```python
from build123d import *

# Parameters (mm, degrees)
SKETCH_1_W      = 13.9
SKETCH_1_H      = 13.9
EXTRUDE_1_DEPTH = 5.5
FILLET_1_R      = 1


with BuildPart() as part:
    # Эскиз1 → Бобышка-Вытянуть1 (new body)
    with BuildSketch(Plane.XY):
        Rectangle(SKETCH_1_W, SKETCH_1_H)
    extrude(amount=EXTRUDE_1_DEPTH)

    # Эскиз3 → Отверстие обработанное метчиком M52 (revolve, cut)
    with BuildSketch(Plane(origin=(0, 0, 5.5), x_dir=(0, -1, 0), z_dir=(1, 0, 0))):
        Polygon((0, 0), (0, 5.5), (2.6, 5.5), (2.1, 5), (2.1, 0.5), (2.6, 0), align=None)
    revolve(axis=Axis((0, 0, 11.85), (0, 0, -1)), mode=Mode.SUBTRACT)

    # Скругление1
    fillet_1_edges = [part.edges().sort_by_distance(p)[0] for p in [
        (6.95, -6.95, 2.75),
        (-6.95, -6.95, 2.75),
        (-6.95, 6.95, 2.75),
        (6.95, 6.95, 2.75),
    ]]
    fillet(fillet_1_edges, radius=FILLET_1_R)


solid = part.part
```
Geometry check sheet. Reference: the model listing, model coordinates, mm. Coordinates: 2 decimals unless noted, no trailing zeros. Order: outer loops, then holes, each group sorted by start corner. A loop starts at its lowest first (then second) coordinate and runs counter-clockwise, first axis right, second up.
Q1. Depth check by flat-ended pin: pin 1 Ø3.5 at (x, y) = (0, 0) entering from -Z. Enter the tip coordinate at first touch or a pass-through.
Reply:
pin 1: passes through
Q2. Sectioned sample at C-C on z = 3.5. Record the cut outline in (x, y).
Reply:
outline: (-6.95, -5.95) arc R1 ccw to (-5.95, -6.95) - (5.95, -6.95) arc R1 ccw to (6.95, -5.95) - (6.95, 5.95) arc R1 ccw to (5.95, 6.95) - (-5.95, 6.95) arc R1 ccw to (-6.95, 5.95) - close; hole circle Ø4.2 at (0, 0)
Q3. Sectioned sample at A-A on y = 0. Record the cut outline in (x, z), and give its area (4 significant figures).
Reply:
outline: (-6.95, 0) - (-2.6, 0) - (-2.1, 0.5) - (-2.1, 5) - (-2.6, 5.5) - (-6.95, 5.5) - close; (2.1, 0.5) - (2.6, 0) - (6.95, 0) - (6.95, 5.5) - (2.6, 5.5) - (2.1, 5) - close
area: 52.85 mm2
Q4. Thickness scan on probe 1 along Y at (x, z) = (0, 2.85); probe 2 along Y at (x, z) = (-1.75, 0.9). Record the ranges inside material, lowest first.
Reply:
probe 1: y = -6.95 to -2.1, 2.1 to 6.95
probe 2: y = -6.95 to -1.16, 1.16 to 6.95
Q5. Draft check along X on faces 1 (the face through (6.95, 0, 3)), 2 (the face through (-0.631, -2.003, 2.782)), 3 (the face through (0, -6.95, 3)). Enter one of: released by +X, released by -X, zero draft, split by the parting line, or undercut.
Reply:
face 1: released by +X
face 2: undercut
face 3: zero draft
